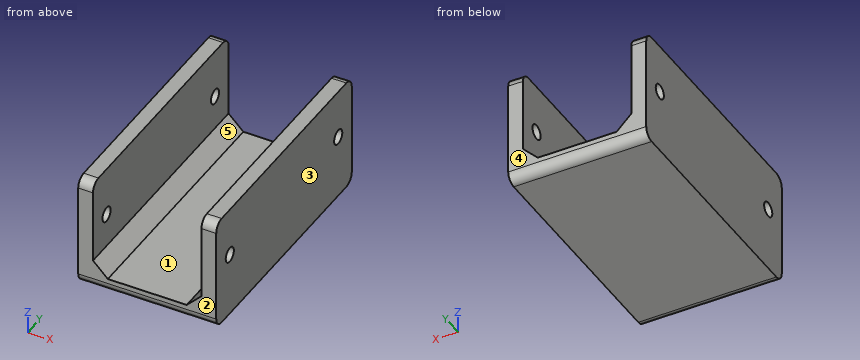
Autodesk Inventor part; units mm, degrees
ref_plane "YZ Plane" through (0, 0, 0) normal (1, 0, 0) x (0, 1, 0)
ref_plane "XZ Plane" through (0, 0, 0) normal (0, 1, 0) x (-1, 0, 0)
ref_plane "XY Plane" through (0, 0, 0) normal (0, 0, 1) x (1, 0, 0)
sketch "Sketch1" plane through (0, 0, 0) normal (0, 1, 0) x (-1, 0, 0)
  line L0 (0, 0) -> (0, -23)
  line L1 (0, -23) -> (-28, -23)
  line L2 (-28, -23) -> (-28, 0)
  line L3 (-28, 0) -> (-25, 0)
  line L4 (-25, 0) -> (-25, -20)
  line L5 (-25, -20) -> (-3, -20)
  line L6 (-3, -20) -> (-3, 0)
  line L7 (-3, 0) -> (0, 0)
  dimension "d0" = 3
  dimension "d1" = 3
  dimension "d2" = 3
  dimension "d3" = 28
  dimension "d4" = 23
extrude "Extrusion1" add sketch "Sketch1" along normal blind 50
sketch "Sketch2" plane through (0, 0, -23) normal (-1, 0, 0) x (0, 0, 1)
  circle A0 centre (13, 45) radius 1.5
  circle A1 centre (13, 5) radius 1.5
  line L0 (23, 0) -> (23, 50) construction
  line L1 (13, 5) -> (13, 45) construction
  line L2 (0, 0) -> (23, 0) construction
  dimension "d8" = 3
  dimension "d9" = 10
  dimension "d11" = 40
  dimension "d12" = 5
extrude "Extrusion2" cut sketch "Sketch2" against normal up to surface (28 mm away)
fillet "Fillet1" radius 2 6 edges at (1.5, 50, 0) (1.5, 0, 0) (26.5, 50, 0) (26.5, 0, 0) (14, 50, -23) (14, 0, -23)
chamfer "Chamfer1" distance 3 angle 45 2 edges at (3, 25, -20) (25, 25, -20)
properties part number "Front_Wheel_Stand"
Verification items for the finished model (mm, model axes). Face numbers are marked on the shaded views. A direction names the side the tool comes from. Give positions to 0.01 mm unless a question says otherwise; leave off trailing zeros. Write each loop counter-clockwise with the first axis right and the second up, starting at its lowest first coordinate (ties: lowest second). Pieces come first, ordered by that corner, then holes.
(1) Cross-section at D-D (x = 20). Enter the section's corners in (y, z).
(2) Cross-section at A-A (z = -10). Enter the section's corners in (x, y).
(3) Cross-section at C-C (y = 45). Enter the section's corners in (x, z), plus the area to 3 significant figures.
(4) Material ranges on line 1 (Y direction, x = 27.4, z = -10); line 2 (X direction, y = 3.5, z = -4.75); line 3 (Z direction, x = 16.75, y = 30), recorded low to high.
(5) Gauge pin test, flat ends, axial feed: pin 1 (3.5 mm diameter, centred on y = 5, z = -10, fed in from +X); pin 2 (6 mm diameter, centred on x = 20, y = 15, fed in from +Z); pin 3 (5 mm diameter, centred on x = 14, y = 16.5, fed in from +Z). Record the tip position at first contact, or that the pin passes through.
(6) Mould release check, pull along X, two halves, no side actions. Record for the marked faces 3, 4 and 5: +X half, -X half, draft (parallel to the pull), parting line (faces both ways), or undercut.
(7) Cross-section at B-B (z = -16.25). Enter the section's corners in (x, y).
(8) Access from +Z, -Z, +X, -X, +Y, -Y to the whole of each face (thin tool, end or side, straight path). Record for the marked faces 1 and 2.
Worked out:
1. outline: (0, -21) arc R2 ccw to (2, -23) - (48, -23) arc R2 ccw to (50, -21) - (50, -20) - (0, -20) - close
2. outline: (0, 0) - (3, 0) - (3, 3.5) - (0, 3.5) - close; (0, 6.5) - (3, 6.5) - (3, 43.5) - (0, 43.5) - close; (0, 46.5) - (3, 46.5) - (3, 50) - (0, 50) - close; (25, 0) - (28, 0) - (28, 3.5) - (25, 3.5) - close; (25, 6.5) - (28, 6.5) - (28, 43.5) - (25, 43.5) - close; (25, 46.5) - (28, 46.5) - (28, 50) - (25, 50) - close
3. outline: (0, -23) - (28, -23) - (28, -11.5) - (25, -11.5) - (25, -17) - (22, -20) - (6, -20) - (3, -17) - (3, -11.5) - (0, -11.5) - close; (0, -8.5) - (3, -8.5) - (3, 0) - (0, 0) - close; (25, -8.5) - (28, -8.5) - (28, 0) - (25, 0) - close
3. area: 195 mm2
4. line 1: y = 0 to 3.5, 6.5 to 43.5, 46.5 to 50
4. line 2: x = 0 to 3, 25 to 28
4. line 3: z = -23 to -20
5. pin 1: stops at x = 28
5. pin 2: stops at z = -19
5. pin 3: stops at z = -20
6. face 3: +X half
6. face 4: draft
6. face 5: undercut
7. outline: (0, 0) - (3, 0) - (3, 50) - (0, 50) - close; (25, 0) - (28, 0) - (28, 50) - (25, 50) - close
8. face 1: +Z, +Y, -Y
8. face 2: +Z, -Z, +X, -X, -Y
